For this review, use the dimensioned drawing (mm, ordinates from the lowest corner) and the shaded views. A direction names the side the tool comes from. Give positions to 0.01 mm unless a question says otherwise; leave off trailing zeros. Write each loop counter-clockwise with the first axis right and the second up, starting at its lowest first coordinate (ties: lowest second). Pieces come first, ordered by that corner, then holes.
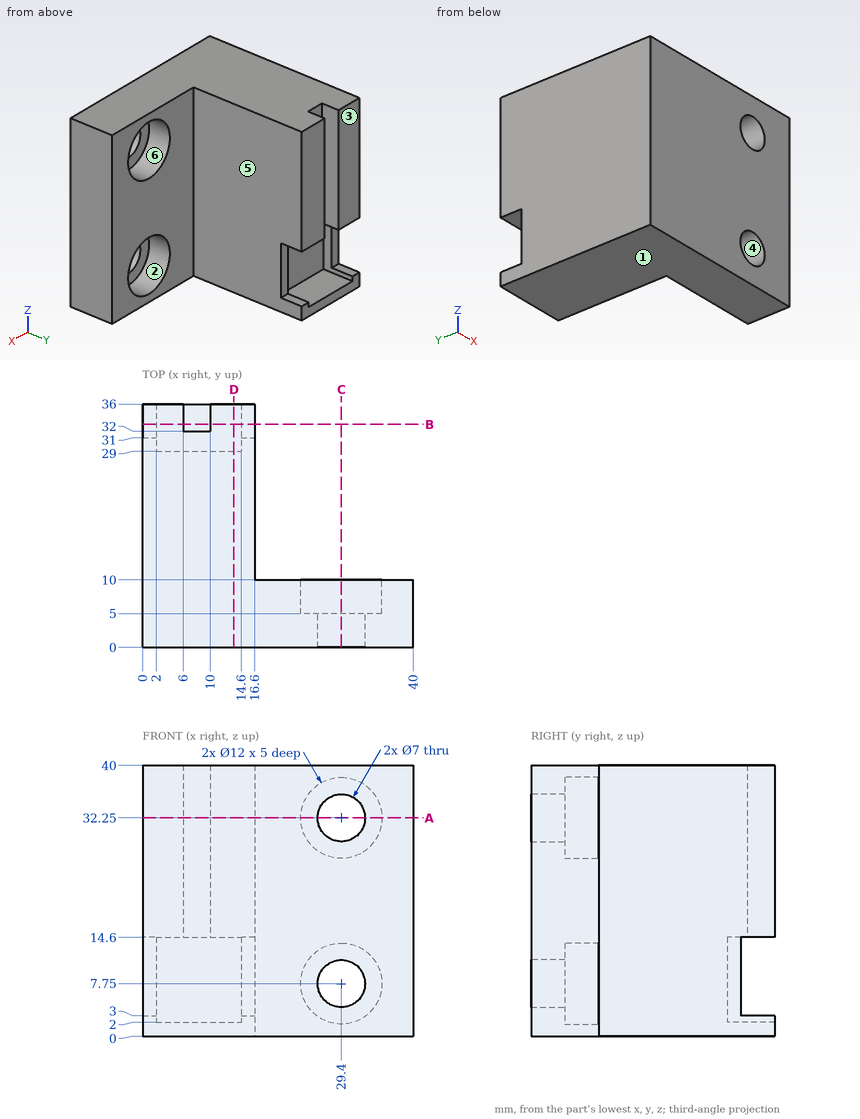
(1) We need section C-C (x = 29.4). Write out the cut boundary in (y, z).
(2) We need section B-B (y = 33). Write out the cut boundary in (x, z).
(3) Tool access review of the marked faces 4, 5 and 6: name each direction out of +Z, -Z, +X, -X, +Y, -Y from which nothing blocks a thin tool from reaching the whole face with its end or side.
(4) Clearance check with flat-ended pins moving along their axes: pin 1 Ø9 at (x, z) = (29.4, 7.75) entering from +Y; pin 2 Ø6 at (x, z) = (26.5, 33.5) entering from +Y; pin 3 Ø6.5 at (x, z) = (29.4, 32.25) entering from -Y (3 decimals); pin 4 Ø2 at (y, z) = (34.5, 22.5) entering from +X. State where each tip first meets the part, or that it passes through.
(5) We need section D-D (x = 13.5). Write out the cut boundary in (y, z).
(6) We need section A-A (z = 32.25). Write out the cut boundary in (x, y), and give its area (3 significant figures).
(7) For L1, parallel to Z at x = 29, y = 7; L2, parallel to X at y = 7, z = 32; L3, parallel to X at y = 21, z = 17.5, list the stretches that pass through material, from the lowest coordinate up.
(8) The part is to be moulded in two halves that separate along Z. For the marked faces 1, 2 and 3, say which applies: +Z half, -Z half, draft (parallel to the pull), parting line (faces both ways), or undercut.
The answers:
1. outline: (0, 0) - (10, 0) - (10, 1.75) - (5, 1.75) - (5, 4.25) - (0, 4.25) - close; (0, 11.25) - (5, 11.25) - (5, 13.75) - (10, 13.75) - (10, 26.25) - (5, 26.25) - (5, 28.75) - (0, 28.75) - close; (0, 35.75) - (5, 35.75) - (5, 38.25) - (10, 38.25) - (10, 40) - (0, 40) - close
2. outline: (0, 0) - (16.6, 0) - (16.6, 3) - (14.6, 3) - (14.6, 2) - (2, 2) - (2, 3) - (0, 3) - close; (0, 14.6) - (6, 14.6) - (6, 40) - (0, 40) - close; (10, 14.6) - (16.6, 14.6) - (16.6, 40) - (10, 40) - close
3. face 4: +Y, -Y
3. face 5: +Z, -Z, +X, +Y
3. face 6: +Y
4. pin 1: stops at y = 5
4. pin 2: stops at y = 10
4. pin 3: passes through
4. pin 4: stops at x = 16.6
5. outline: (0, 0) - (36, 0) - (36, 2) - (29, 2) - (29, 14.6) - (36, 14.6) - (36, 40) - (0, 40) - close
6. outline: (0, 0) - (25.9, 0) - (25.9, 5) - (23.4, 5) - (23.4, 10) - (16.6, 10) - (16.6, 36) - (10, 36) - (10, 32) - (6, 32) - (6, 36) - (0, 36) - close; (32.9, 0) - (40, 0) - (40, 10) - (35.4, 10) - (35.4, 5) - (32.9, 5) - close
6. area: 721 mm2
7. L1: z = 0 to 1.76, 13.74 to 26.26, 38.24 to 40
7. L2: x = 0 to 23.41, 35.39 to 40
7. L3: x = 0 to 16.6
8. face 1: -Z half
8. face 2: undercut
8. face 3: draft
